Autodesk Inventor part; units mm, degrees
ref_plane "YZ Plane" through (0, 0, 0) normal (1, 0, 0) x (0, 1, 0)
ref_plane "XZ Plane" through (0, 0, 0) normal (0, 1, 0) x (-1, 0, 0)
ref_plane "XY Plane" through (0, 0, 0) normal (0, 0, 1) x (1, 0, 0)
sketch "Sketch1" plane through (0, 0, 0) normal (0, 0, 1) x (1, 0, 0)
  line L0 (0, 0) -> (118, 0)
  line L1 (118, 0) -> (118, 15)
  line L2 (118, 15) -> (0, 15)
  line L3 (0, 15) -> (0, 0)
  dimension "d0" = 118
  dimension "d1" = 15
extrude "Extrusion1" add sketch "Sketch1" along normal blind 8
sketch "Sketch2" plane through (0, 0, 8) normal (0, 0, 1) x (1, 0, 0)
  circle A0 centre (14, 5) radius 1.6
  circle A1 centre (44, 5) radius 1.6
  circle A2 centre (74, 5) radius 1.6
  line L0 (0, 15) -> (0, 0)
  line L1 (118, 0) -> (118, 15)
  line L2 (0, 0) -> (118, 0)
  circle A3 centre (104, 5) radius 1.5
  line L3 (118, 15) -> (0, 15)
  circle A4 centre (29, 10) radius 1.5
  circle A5 centre (89, 10) radius 1.5
  point P0 (59, 0)
  dimension "d4" = 3.2
  dimension "d5" = 3.2
  dimension "d6" = 3.2
  dimension "d11" = 5
  dimension "d14" = 3
  dimension "d15" = 30
  dimension "d16" = 30
  dimension "d17" = 30
  dimension "d18" = 14
  dimension "d19" = 14
  dimension "d20" = 3
  dimension "d21" = 3
  dimension "d22" = 5
  dimension "d23" = 29
  dimension "d24" = 29
extrude "Extrusion2" cut sketch "Sketch2" against normal blind 10 contours A0 | A1 | A2 | A3 | A4 | A5
sketch "Sketch3" plane through (0, 0, 8) normal (0, 0, 1) x (1, 0, 0)
  circle A0 centre (44, 5) radius 1.6
  circle A1 centre (104, 5) radius 1.5
  circle A2 centre (14, 5) radius 1.6
  circle A3 centre (74, 5) radius 1.6
  arc A4 (19, 7.4135) -> (17, 9.4135) centre (17, 7.4135) ccw
  line L0 (17, 9.4135) -> (11, 9.4135)
  arc A5 (11, 9.4135) -> (9, 7.4135) centre (11, 7.4135) ccw
  line L1 (9, 7.4135) -> (9, -0.5865)
  arc A6 (19, -0.5865) -> (9, -0.5865) centre (14, -8.0699) ccw
  line L2 (19, -0.5865) -> (19, 7.4135)
  circle A7 centre (14, 5) radius 1.6
  arc A8 (49, 7.4135) -> (47, 9.4135) centre (47, 7.4135) ccw
  line L3 (47, 9.4135) -> (41, 9.4135)
  arc A9 (41, 9.4135) -> (39, 7.4135) centre (41, 7.4135) ccw
  line L4 (39, 7.4135) -> (39, -0.5865)
  arc A10 (49, -0.5865) -> (39, -0.5865) centre (44, -8.0699) ccw
  line L5 (49, -0.5865) -> (49, 7.4135)
  circle A11 centre (44, 5) radius 1.6
  arc A12 (79, 7.4135) -> (77, 9.4135) centre (77, 7.4135) ccw
  line L6 (77, 9.4135) -> (71, 9.4135)
  arc A13 (71, 9.4135) -> (69, 7.4135) centre (71, 7.4135) ccw
  line L7 (69, 7.4135) -> (69, -0.5865)
  arc A14 (79, -0.5865) -> (69, -0.5865) centre (74, -8.0699) ccw
  line L8 (79, -0.5865) -> (79, 7.4135)
  circle A15 centre (74, 5) radius 1.6
  arc A16 (109, 7.4135) -> (107, 9.4135) centre (107, 7.4135) ccw
  line L9 (107, 9.4135) -> (101, 9.4135)
  arc A17 (101, 9.4135) -> (99, 7.4135) centre (101, 7.4135) ccw
  line L10 (99, 7.4135) -> (99, -0.5865)
  arc A18 (109, -0.5865) -> (99, -0.5865) centre (104, -8.0699) ccw
  line L11 (109, -0.5865) -> (109, 7.4135)
  circle A19 centre (104, 5) radius 1.6
  line L12 (9, -0.5865) -> (19, -0.5865)
  line L13 (39, -0.5865) -> (49, -0.5865)
  line L14 (69, -0.5865) -> (79, -0.5865)
  line L15 (99, -0.5865) -> (109, -0.5865)
extrude "Extrusion3" cut sketch "Sketch3" against normal blind 3 contours A1 | L2 A6 L1 A5 L0 A4 | L12 A6 | L5 A10 L4 A9 L3 A8 | L13 A10 | L8 A14 L7 A13 L6 A12 | L14 A14 | L11 A18 L10 A17 L9 A16 | L15 A18 | A19
equation "\"d15\" = d16"
equation "\"d16\" = d17"
equation "\"d18\" = d19"
equation "\"d23\" = d24"
equation "\"d24\" = d19 + 0.5 * d15"
properties part number "brush rack holder"
Check sheet for the modelled part. Datum: model origin and axes. Units: mm. A direction names the side the tool comes from. Give positions to 0.01 mm unless a question says otherwise; leave off trailing zeros. Order: outer loops, then holes, each group sorted by start corner. A loop starts at its lowest first (then second) coordinate and runs counter-clockwise, first axis right, second up. Notation, with made-up numbers: M 30.5,-7.75 L 70.5,-7.75 A25 cw 70.5,6.25 Z; hole C -24.75,73.25 d6. An arc over 180 degrees is marked long. Answer in a Markdown table with one row per item.
1) Thickness scan on L1, parallel to X at y = 5.25, z = 1.75; L2, parallel to X at y = 2.25, z = 5.5; L3, parallel to X at y = 10.25, z = 2.5. Record the ranges inside material, lowest first. Write a range as [from, to].
Filled sheet:
| item | result |
|---|---|
| L1 | x = [0, 12.42], [15.58, 42.42], [45.58, 72.42], [75.58, 102.52], [105.48, 118] |
| L2 | x = [0, 9], [19, 39], [49, 69], [79, 99], [109, 118] |
| L3 | x = [0, 27.52], [30.48, 87.52], [90.48, 118] |
2) Cross-section at C-C, the plane x = 104. Enter the section's corners in (y, z), plus the area to 3 significant figures.
Filled sheet:
| item | result |
|---|---|
| outline | M 0,0 L 3.5,0 L 3.5,5 L 0,5 Z; M 6.5,0 L 15,0 L 15,8 L 9.41,8 L 9.41,5 L 6.5,5 Z |
| area | 76.8 mm2 |
3) Gauge pin test, flat ends, axial feed: P1, Ø1.5, axis at y = 5, z = 6.5, coming from the -X side; P2, Ø4.5, axis at x = 41.5, y = 5.5, coming from the +Z side; P3, Ø0.9, axis at x = 43.5, z = 6, coming from the -Y side. Record the tip position at first contact, or that the pin passes through.
Filled sheet:
| item | result |
|---|---|
| P1 | stops at x = 0 |
| P2 | stops at z = 5 |
| P3 | stops at y = 9.41 |
4) Cross-section at A-A, the plane x = 14. Enter the section's corners in (y, z).
Filled sheet:
| item | result |
|---|---|
| outline | M 0,0 L 3.4,0 L 3.4,5 L 0,5 Z; M 6.6,0 L 15,0 L 15,8 L 9.41,8 L 9.41,5 L 6.6,5 Z |
5) Access from +Z, -Z, +X, -X, +Y, -Y to the whole of each face (thin tool, end or side, straight path). Record for faces 5 (the cylindrical face through (44.74, 3.58, 2.54)), 6 (the cylindrical face through (99.6, 8.84, 6.52)).
Filled sheet:
| item | result |
|---|---|
| face 5 | +Z, -Z |
| face 6 | +Z, -Y |
6) Cross-section at B-B, the plane y = 2.25. Enter the section's corners in (x, z).
Filled sheet:
| item | result |
|---|---|
| outline | M 0,0 L 118,0 L 118,8 L 109,8 L 109,5 L 99,5 L 99,8 L 79,8 L 79,5 L 69,5 L 69,8 L 49,8 L 49,5 L 39,5 L 39,8 L 19,8 L 19,5 L 9,5 L 9,8 L 0,8 Z |
7) Cross-section at D-D, the plane x = 29. Enter the section's corners in (y, z).
Filled sheet:
| item | result |
|---|---|
| outline | M 0,0 L 8.5,0 L 8.5,8 L 0,8 Z; M 11.5,0 L 15,0 L 15,8 L 11.5,8 Z |
8) Release check for a two-part mould opening along X. For faces 1 (the flat face through (44, 9.414, 7)), 2 (the flat face through (118, 7, 4)), 3 (the cylindrical face through (27.5, 10.07, 4.06)), 4 (the flat face through (0, 8, 4)) record: +X half, -X half, draft (parallel to the pull), parting line (faces both ways), or undercut.
Filled sheet:
| item | result |
|---|---|
| face 1 | undercut |
| face 2 | +X half |
| face 3 | undercut |
| face 4 | -X half |
